Autodesk Inventor part; units mm, degrees
ref_plane "YZ Plane" through (0, 0, 0) normal (1, 0, 0) x (0, 1, 0)
ref_plane "XZ Plane" through (0, 0, 0) normal (0, 1, 0) x (-1, 0, 0)
ref_plane "XY Plane" through (0, 0, 0) normal (0, 0, 1) x (1, 0, 0)
sketch "Boceto1" plane through (0, 0, 0) normal (0, 0, 1) x (1, 0, 0)
  line L0 (200.6138, -49.1011) -> (347.0892, -49.1011)
  line L1 (366.6054, -71.1) -> (366.6054, -332.1)
  line L2 (352.0892, -357.1011) -> (151.6064, -357.1011)
  line L3 (124.6054, -332.1) -> (124.6054, -152.9933)
  line L4 (366.6054, -332.1) -> (366.6054, -357.1011)
  line L5 (352.0892, -357.1011) -> (366.6054, -357.1011)
  line L6 (347.0892, -49.1011) -> (366.6054, -49.1011)
  line L7 (366.6054, -71.1) -> (366.6054, -49.1011)
  line L8 (151.6064, -357.1011) -> (124.6054, -357.1011)
  line L9 (124.6054, -332.1) -> (124.6054, -357.1011)
  line L10 (200.6138, -49.1011) -> (185.295, -49.1011)
  arc A0 (185.295, -49.1011) -> (124.6054, -152.9933) centre (292.3571, -181.3147) ccw
  dimension "d2" = 308
  dimension "d3" = 242
extrude "Extrusión2" add sketch "Boceto1" along normal blind 2
fillet "Empalme1" radius 25 3 edges at (366.6054, -49.1011, 1) (366.6054, -357.1011, 1) (124.6054, -357.1011, 1)
sketch "Boceto3" plane through (0, 0, 2) normal (0, 0, 1) x (1, 0, 0)
  line L0 (341.6054, -357.1011) -> (149.6054, -357.1011)
  line L1 (366.6054, -74.1011) -> (366.6054, -332.1011)
  line L2 (185.295, -49.1011) -> (341.6054, -49.1011)
  line L3 (124.6054, -332.1011) -> (124.6054, -152.9933)
  circle A0 centre (164.6054, -354.1011) radius 1.75
  circle A1 centre (326.6054, -354.1011) radius 1.75
  circle A2 centre (127.6054, -196.1011) radius 1.75
  circle A3 centre (363.6054, -307.1011) radius 1.75
  circle A4 centre (363.6054, -99.1011) radius 1.75
  circle A5 centre (245.1054, -52.1011) radius 1.75
  point P0 (200.6138, -49.1011)
  point P1 (0, 0)
  dimension "d7" = 3.5
  dimension "d8" = 3.5
  dimension "d9" = 3.5
  dimension "d10" = 3.5
  dimension "d11" = 3.5
  dimension "d12" = 3.5
  dimension "d13" = 3
  dimension "d14" = 3
  dimension "d15" = 3
  dimension "d16" = 3
  dimension "d17" = 3
  dimension "d18" = 3
  dimension "d19" = 121.5
  dimension "d20" = 161
  dimension "d21" = 50
  dimension "d22" = 50
  dimension "d23" = 40
  dimension "d24" = 40
extrude "Extrusión3" cut sketch "Boceto3" against normal blind 2
fillet "Empalme2" radius 20 1 edges at (185.295, -49.1011, 1)
fillet "Empalme3" radius 100 1 edges at (124.6054, -152.9933, 1)
equation "\"d14\" = d13"
equation "\"d15\" = d13"
equation "\"d16\" = d13"
equation "\"d17\" = d13"
equation "\"d18\" = d13"
properties part number "metacrilat proteccio dret"
Verification items for the finished model (mm, model axes). Round coordinates to 2 decimals unless told otherwise and drop trailing zeros. Write each question's results on one line, items separated by ' | '. Start each with the question number.
1. Depth check by flat-ended pin: P1, Ø5.5, axis at x = 326.61, y = -354.1, coming from the -Z side. Enter the tip coordinate at first touch or a pass-through.
2. Material ranges on probe 1 along Y at (x, z) = (177, 0.25); probe 2 along X at (y, z) = (-129, 0.2); probe 3 along Y at (x, z) = (172.5, 1.35), recorded low to high. Write a range as from..to.
3. Cross-section at A-A (z = 1.6). Count the separate pieces of the cut face and the enclosed holes in it, then the cut area to 3 significant figures.
Solutions:
1) P1: stops at z = 0
2) probe 1: y = -357.1..-56.27 | probe 2: x = 130.47..366.61 | probe 3: y = -357.1..-60.58
3) separate pieces: 1 | enclosed holes: 6 | area: 71,800 mm2
